Could you check a few things on this model? Use its own coordinates, in mm. Round coordinates to 2 decimals unless told otherwise and drop trailing zeros. Write each loop counter-clockwise with the first axis right and the second up, starting at its lowest first coordinate (ties: lowest second). Pieces come first, ordered by that corner, then holes. Notation, with made-up numbers: (47, 81) -> (74, 81) arc R26 cw to (74, 97) -> close; hole circle Ø1 at (27.5, 75). An arc over 180 degrees is marked (long way). One line per question, with ' | ' between items. Start each with the question number.
1. Imagine slicing it at B-B, the plane x = 54. List the corners of the cut face in (y, z) for me, and give its area (3 significant figures).
2. Thinking about a two-plate mould opening in Y: for faces 1 (the cylindrical face through (-9.764, 74.362, 2.465)), 2 (the cylindrical face through (-68.425, -13.117, 2.535)), 3 (the flat face through (-1, 1, 5)), which applies, released by +Y, released by -Y, zero draft, split by the parting line, or undercut?
3. Imagine slicing it at C-C, the plane y = -42. List the corners of the cut face in (x, z) for me.
4. If I drill on line 1 along X through (y, z) = (22, 1.9); line 2 along X through (y, z) = (-34.5, 4.3); line 3 along Y through (x, z) = (-63, 2), over which ranges is the centre line in solid material (lowest first)? Write a range as [from, to].
5. Imagine slicing it at A-A, the plane z = 2.7. List the corners of the cut face in (x, y) for me, and give its area (3 significant figures).
6. For pin 1 Ø1.5 at (x, z) = (32, 0.5) entering from +Y; pin 2 Ø1 at (x, z) = (-45.5, 1) entering from -Y; pin 3 Ø4.5 at (x, y) = (70.29, 11.35) entering from -Z; pin 4 Ø2 at (y, z) = (-37, 3) entering from +X, each with a flat end and sliding along its axis, tell me the tip position at first contact or that it passes through.
from build123d import *

# Parameters (mm, degrees)
F0_R       = 75
F1_DEPTH   = 5
F5_D       = 5
F5_ON_F2_D = 5


with BuildPart() as f1:
    # F0 (on Top) → F1 (new body)
    with BuildSketch(Plane.XY):
        Circle(F0_R)
    extrude(amount=F1_DEPTH)

    # F3: F1 across plane


with BuildPart() as f1_1:
    add(f1.part)
    add(f1.part.mirror(Plane.YZ))

    # F5 (through all)
    with Locations(Plane(origin=(0, 0, 0), x_dir=(1, 0, 0), z_dir=(0, 0, -1))):
        with Locations((-70.9224045277, -9.4928164221), (-70.9224045277, 13.0071835779)):
            Hole(F5_D / 2)

    # F5 on F2 (through all)
    with Locations(Plane(origin=(0, 0, 0), x_dir=(1, 0, 0), z_dir=(0, 0, -1))):
        with Locations((70.2925920486, -11.3482945785), (70.2925920486, 11.1517054215)):
            Hole(F5_ON_F2_D / 2)


solid = f1_1.part
Geometry results:
1) outline: (-52.05, 0) -> (52.05, 0) -> (52.05, 5) -> (-52.05, 5) -> close | area: 520 mm2
2) face 1: split by the parting line | face 2: undercut | face 3: zero draft
3) outline: (-62.14, 0) -> (62.14, 0) -> (62.14, 5) -> (-62.14, 5) -> close
4) line 1: x = [-71.7, 71.7] | line 2: x = [-66.59, 66.59] | line 3: y = [-40.69, 40.69]
5) outline: circle Ø150 at (0, 0); hole circle Ø5 at (-70.92, -13.01); hole circle Ø5 at (-70.92, 9.49); hole circle Ø5 at (70.29, -11.15); hole circle Ø5 at (70.29, 11.35) | area: 17,600 mm2
6) pin 1: stops at y = 68.18 | pin 2: stops at y = -60 | pin 3: passes through | pin 4: stops at x = 65.8
